Check sheet for the drawn part. Datum: minimum x, y, z corner. Units: mm. A direction names the side the tool comes from. Give positions to 0.01 mm unless a question says otherwise; leave off trailing zeros. Loops run counter-clockwise (first coordinate to the right, second up) from the corner with the lowest first, then second, coordinate; pieces in that order, holes last. Notation, with made-up numbers: (46.25, 41.5) - (72.25, 41.5) arc R16 cw to (72.25, 63.5) - close; hole circle Ø11 at (38.25, 4.5). An arc over 180 degrees is marked (long way). One line per item, written item: value. Start each with the question number.
1. Access from +Z, -Z, +X, -X, +Y, -Y to the whole of each face (thin tool, end or side, straight path). Record for the marked faces 1 and 2.
2. Sectioned sample at A-A (x = 7.75). Record the cut outline in (y, z) (1 decimal).
3. Sectioned sample at D-D (x = 2). Record the cut outline in (y, z) (1 decimal).
4. Gauge pin test, flat end, axial feed: pin 1 (1.6 mm diameter, centred on y = 13, z = 1, fed in from +X). Record the tip position at first contact, or that the pin passes through.
5. Mould release check, pull along Y, two halves, no side actions. Record for the marked faces 3, 4 and 5: pulls with the +Y half, pulls with the -Y half, needs draft (parallel to the pull), parting line crosses it, or undercut.
6. Scan lines: L1, parallel to Z at x = 8.25, y = 21 (1 decimal); L2, parallel to X at y = 21.5, z = 0.35; L3, parallel to Y at x = 16.25, z = 1.4. Record each from-to range of solid material in increasing order. Write a range as [from, to].
7. Sectioned sample at C-C (z = 1.25). Record the cut outline in (x, y).
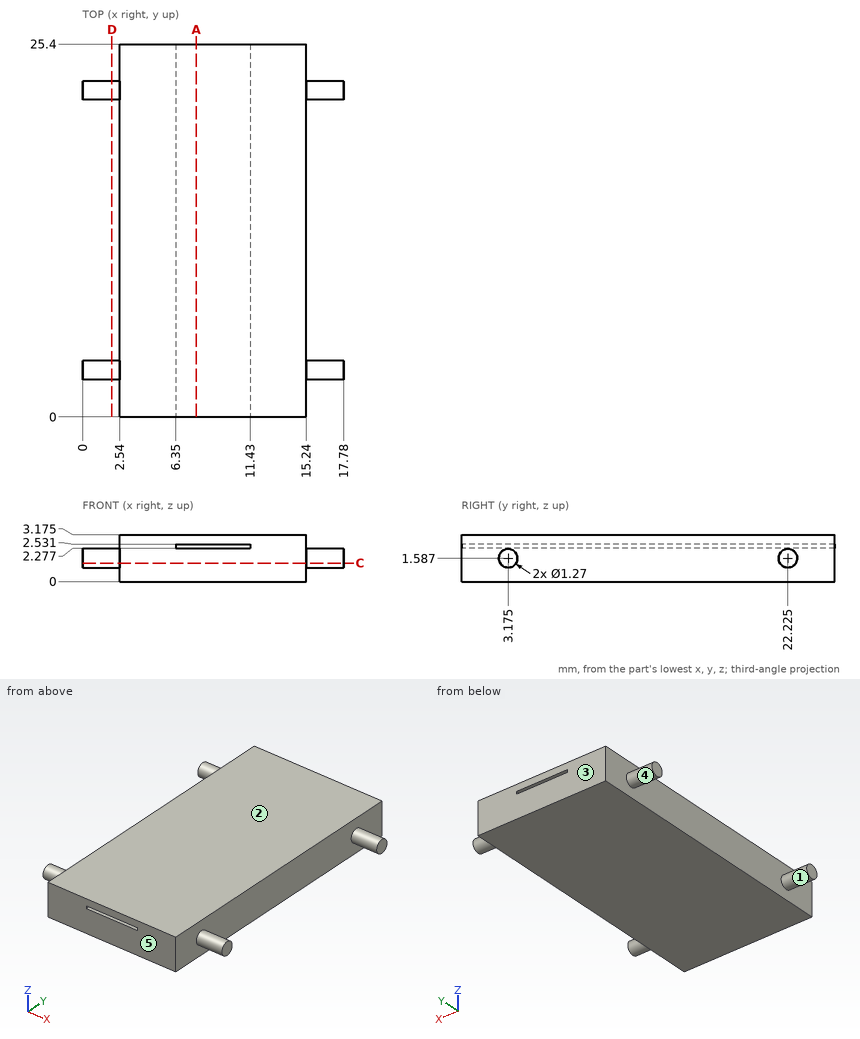
Results are:
1. face 1: -X
1. face 2: +Z, +X, -X, +Y, -Y
2. outline: (0, 0) - (25.4, 0) - (25.4, 2.3) - (0, 2.3) - close; (0, 2.5) - (25.4, 2.5) - (25.4, 3.2) - (0, 3.2) - close
3. outline: circle Ø1.3 at (3.2, 1.6); circle Ø1.3 at (22.2, 1.6)
4. pin 1: stops at x = 15.24
5. face 3: pulls with the +Y half
5. face 4: undercut
5. face 5: pulls with the -Y half
6. L1: z = [0, 2.3], [2.5, 3.2]
6. L2: x = [2.54, 15.24]
6. L3: y = [2.57, 3.78], [21.62, 22.83]
7. outline: (0, 2.64) - (2.54, 2.64) - (2.54, 0) - (15.24, 0) - (15.24, 2.64) - (17.78, 2.64) - (17.78, 3.71) - (15.24, 3.71) - (15.24, 21.69) - (17.78, 21.69) - (17.78, 22.76) - (15.24, 22.76) - (15.24, 25.4) - (2.54, 25.4) - (2.54, 22.76) - (0, 22.76) - (0, 21.69) - (2.54, 21.69) - (2.54, 3.71) - (0, 3.71) - close
